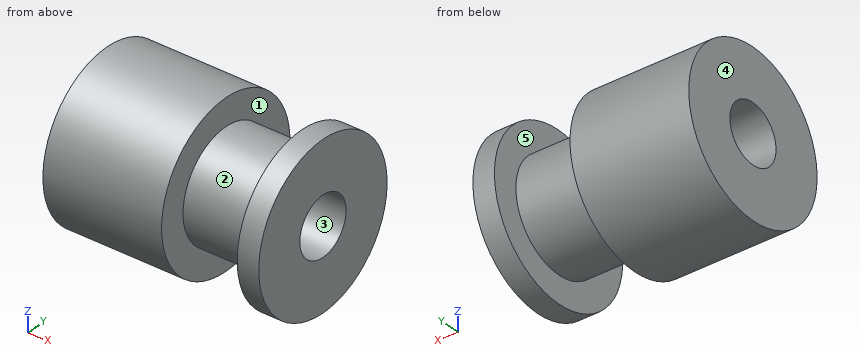
Autodesk Inventor part; units mm, degrees
ref_plane "YZ Plane" through (0, 0, 0) normal (1, 0, 0) x (0, 1, 0)
ref_plane "XZ Plane" through (0, 0, 0) normal (0, 1, 0) x (-1, 0, 0)
ref_plane "XY Plane" through (0, 0, 0) normal (0, 0, 1) x (1, 0, 0)
sketch "Sketch1" plane through (0, 0, 0) normal (0, 1, 0) x (-1, 0, 0)
  line L0 (0, 0) -> (0, -7.5)
  line L1 (0, -7.5) -> (2, -7.5)
  line L2 (2, -7.5) -> (2, -5)
  line L3 (2, -5) -> (9, -5)
  line L4 (9, -5) -> (9, -7.5)
  line L5 (9, -7.5) -> (20, -7.5)
  line L6 (20, -7.5) -> (20, 0)
  line L7 (20, 0) -> (0, 0)
  line L8 (0, -2.7) -> (20, -2.7)
  dimension "d0" = 7.5
  dimension "d1" = 7.5
  dimension "d2" = 5
  dimension "d3" = 2
  dimension "d4" = 11
  dimension "d5" = 7
  dimension "d7" = 2.7
revolve "Revolution1" add sketch "Sketch1" angle 360 about axis through (-20, 0, 0) along (1, 0, 0) contours L8 L6 L5 L4 L3 L2 L1 L0
equation "\"d1\" = d0"
properties part number "IdlerPulley"
Can you work these out from the model? Positions are in its coordinate system, mm. Face numbers are marked on the shaded views. A direction names the side the tool comes from. Coordinates: 2 decimals unless noted, no trailing zeros. Write each loop counter-clockwise with the first axis right and the second up, starting at its lowest first coordinate (ties: lowest second). Pieces come first, ordered by that corner, then holes. Notation, with made-up numbers: (86.25, -17) -> (143.25, -17) arc R20 cw to (143.25, -6) -> close; hole circle Ø6 at (47, 68). An arc over 180 degrees is marked (long way). Write item = value, one per line.
(1) On a 3-axis mill with a long thin cutter (end or side, diameter ignored), from which of +Z, -Z, +X, -X, +Y, -Y can I reach the whole of each face in a straight line? I mean the marked faces 4 and 5. Say none if no direction works.
Verdict:
face_4 = +Z, -Z, -X, +Y, -Y
face_5 = none
(2) Imagine slicing it at D-D (y = 3). Please give me the cut outline in (x, z), and give its area (3 significant figures).
Verdict:
outline = (-20, -6.87) -> (-9, -6.87) -> (-9, -4) -> (-2, -4) -> (-2, -6.87) -> (0, -6.87) -> (0, 6.87) -> (-2, 6.87) -> (-2, 4) -> (-9, 4) -> (-9, 6.87) -> (-20, 6.87) -> close
area = 235 mm^2
(3) Thinking about a two-plate mould opening in Z: for the marked faces 1, 2 and 3, which applies, +Z half, -Z half, draft (parallel to the pull), parting line (faces both ways), or undercut?
Verdict:
face_1 = draft
face_2 = parting line
face_3 = undercut
(4) Imagine slicing it at A-A (z = 0). Please give me the cut outline in (x, y).
Verdict:
outline = (-20, -7.5) -> (-9, -7.5) -> (-9, -5) -> (-2, -5) -> (-2, -7.5) -> (0, -7.5) -> (0, -2.7) -> (-20, -2.7) -> close; (-20, 2.7) -> (0, 2.7) -> (0, 7.5) -> (-2, 7.5) -> (-2, 5) -> (-9, 5) -> (-9, 7.5) -> (-20, 7.5) -> close
(5) For pin 1 (3 mm diameter, centred on x = -8.5, z = 3, fed in from -Y); pin 2 (1.5 mm diameter, centred on x = -11.5, z = 4, fed in from -Y), each with a flat end and sliding along its axis, tell me the tip position at first contact or that it passes through.
Verdict:
pin_1 = -7.33
pin_2 = -6.76
(6) If I drill on probe 1 along Y at (x, z) = (-14.75, 0); probe 2 along X at (y, z) = (-3.75, 5.75); probe 3 along Y at (x, z) = (-6.5, 0), over which ranges is the centre line in solid material (lowest first)?
Verdict:
probe_1 = -7.5 to -2.7, 2.7 to 7.5
probe_2 = -20 to -9, -2 to 0
probe_3 = -5 to -2.7, 2.7 to 5
(7) Imagine slicing it at C-C (x = -12.75). Please give me the cut outline in (y, z).
Verdict:
outline = circle Ø15 at (0, 0); hole circle Ø5.4 at (0, 0)
